Read the model definition and answer for the solid it produces. Units are mm, in the model's axes. Face numbers are marked on the shaded views. A direction names the side the tool comes from. Coordinates: 2 decimals unless noted, no trailing zeros. Loops run counter-clockwise (first coordinate to the right, second up) from the corner with the lowest first, then second, coordinate; pieces in that order, holes last. Notation, with made-up numbers: M 89.5,41.25 L 124.5,41.25 A21 cw 124.5,56.25 Z; hole C 73,-31 d11. An arc over 180 degrees is marked long. One line per item, written item: value. Start each with the question number.
1. The part is cut by section D-D (x = -4). Write down the section's boundary in (y, z), then the cut area to 3 significant figures.
2. The part is cut by section C-C (y = -1). Write down the section's boundary in (x, z).
3. The part is cut by section A-A (y = 8). Write down the section's boundary in (x, z), then the cut area to 3 significant figures.
4. Flat-ended cylindrical pins translate along their axes: pin 1 (1 mm diameter, centred on x = 7.5, z = 5, fed in from -Y); pin 2 (1.8 mm diameter, centred on x = 0, y = -20, fed in from -Z); pin 3 (5 mm diameter, centred on x = 6.5, z = 4, fed in from +Y); pin 4 (1.8 mm diameter, centred on x = 0.5, z = 4, fed in from +Y). Find the tip coordinate at first contact, or state that the pin passes through.
5. The part is cut by section B-B (z = 5). State how many separate pieces and enclosed holes the cut face has, then the cut area to 3 significant figures.
6. Determine the mould class of the marked faces 5, 6 and 7 for opening direction Z: +Z half, -Z half, draft (parallel to the pull), parting line (faces both ways), or undercut.
7. For the marked faces 1, 2, 3 and 4, determine the directions among +Z, -Z, +X, -X, +Y, -Y from which every point of the face is accessible in a straight line to the end or side of a thin tool.
8. Consider probe 1 along Z at (x, y) = (7.5, -5); probe 2 along Y at (x, z) = (0, 1.5); probe 3 along Z at (x, y) = (0, -14.25). Determine where each line is inside the solid, lowest interval first.
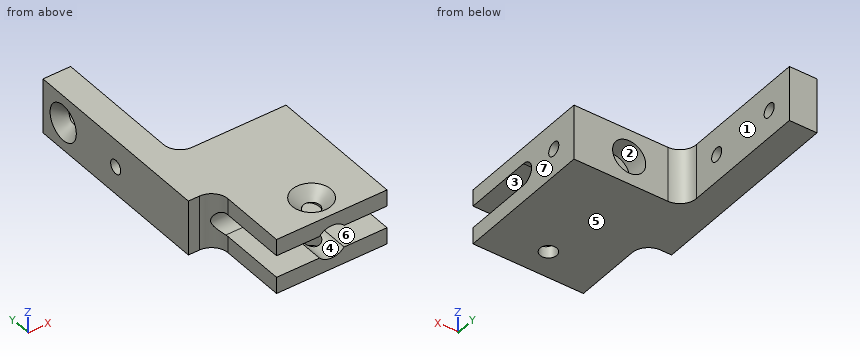
```python
from build123d import *

# Parameters (mm, degrees)
F0_R      = 1.5
F1_DEPTH  = 10
F3_DEPTH  = 25.001001
F4_R      = 1.25
F5_DEPTH  = 25.001001
F6_R      = 1
F7_DEPTH  = 25.001
F6_R_2    = 3
F8_DEPTH  = 4
F2_R      = 1.25
F9_DEPTH  = 10
F10_SIZE  = 2
F11_R     = 3
F12_DEPTH = 17


with BuildPart() as f1:
    # F0 (on Top) → F1 (new body)
    with BuildSketch(Plane.XY):
        Polygon((10.000001, -25), (10.000001, 0), (-7, 0), (-10, 0), (-10, 3), (-10, 26), (-15, 26), (-15, -10), (-13, -10), (-10, -10), (-10, -13), (-10, -25), align=None)
        with Locations((0, -20)):
            Circle(F0_R, mode=Mode.SUBTRACT)
        with BuildLine():
            ThreePointArc((-13, -10), (-10.87868, -10.87868), (-10, -13))
            Line((-10, -13), (-10, -10))
            Line((-10, -10), (-13, -10))
        make_face()
        with BuildLine():
            Line((-10, 0), (-7, 0))
            ThreePointArc((-7, 0), (-9.12132, 0.87868), (-10, 3))
            Line((-10, 3), (-10, 0))
        make_face()
    extrude(amount=F1_DEPTH)

    # F2 (on face) → F3 (cut, through all)
    with BuildSketch(Plane.YZ.offset(10.000001)):
        with BuildLine():
            Line((-12.5, 7), (-25, 7))
            Line((-25, 7), (-25, 3))
            Line((-25, 3), (-12.5, 3))
            ThreePointArc((-12.5, 3), (-10.5, 5), (-12.5, 7))
        make_face()
    extrude(amount=-F3_DEPTH, mode=Mode.SUBTRACT)

    # F4 (on face) → F5 (cut, through all)
    with BuildSketch(Plane(origin=(-15, 0, 0), x_dir=(0, -1, 0), z_dir=(-1, 0, 0))):
        with Locations((-8, 5)):
            Circle(F4_R)
        with Locations((-21, 5)):
            Circle(F4_R)
    extrude(amount=-F5_DEPTH, mode=Mode.SUBTRACT)

    # F6 (on face) → F7 (cut, through all)
    with BuildSketch(Plane(origin=(0, 0, 0), x_dir=(-1, 0, 0), z_dir=(0, 1, 0))):
        with Locations((0, 5)):
            Circle(F6_R)
    extrude(amount=-F7_DEPTH, mode=Mode.SUBTRACT)

    # F6 (on face) → F8 (cut)
    with BuildSketch(Plane(origin=(0, 0, 0), x_dir=(-1, 0, 0), z_dir=(0, 1, 0))):
        with Locations((0, 5)):
            Circle(F6_R_2)
        with Locations((0, 5)):
            Circle(F6_R, mode=Mode.SUBTRACT)
    extrude(amount=-F8_DEPTH, mode=Mode.SUBTRACT)

    # F2 (on face) → F9 (cut)
    with BuildSketch(Plane.YZ.offset(10.000001)):
        with Locations((-5, 5)):
            Circle(F2_R)
    extrude(amount=-F9_DEPTH, mode=Mode.SUBTRACT)

    # F10
    f10_edges = [f1.edges().sort_by_distance(p)[0] for p in [
        (-1.5, -20, 10),
        (-15, 22.25, 5),
    ]]
    chamfer(f10_edges, length=F10_SIZE)

    # F11 (on face) → F12 (cut)
    with BuildSketch(Plane.XZ.offset(25)):
        with Locations((0, 5)):
            Circle(F11_R)
    extrude(amount=-F12_DEPTH, mode=Mode.SUBTRACT)


solid = f1.part
```
Answer block:
1. outline: M -25,0 L 0,0 L 0,10 L -25,10 L -25,7 L -12.5,7 A2 cw -12.5,3 L -25,3 Z
1. area: 194 mm2
2. outline: M -15,0 L 10,0 L 10,10 L -15,10 Z; hole C 0,5 d6
3. outline: M -15,0 L -10,0 L -10,3.75 L -15,3.75 Z; M -15,6.25 L -10,6.25 L -10,10 L -15,10 Z
3. area: 37.5 mm2
4. pin 1: stops at y = -10.56
4. pin 2: passes through
4. pin 3: stops at y = 0
4. pin 4: stops at y = -4
5. separate pieces: 5
5. enclosed holes: 0
5. area: 295 mm2
6. face 5: -Z half
6. face 6: undercut
6. face 7: draft
7. face 1: +Z, -Z, +X, +Y
7. face 2: +Y
7. face 3: +X, -X, -Y
7. face 4: -Y
8. probe 1: z = 0 to 3.75, 6.25 to 10
8. probe 2: y = -25 to -21.5, -18.5 to 0
8. probe 3: z = 0 to 2, 8 to 10
